Design review of the part built by this model. Coordinates are the model's own, in mm. A direction names the side the tool comes from. Give positions to 0.01 mm unless a question says otherwise; leave off trailing zeros. Loops run counter-clockwise (first coordinate to the right, second up) from the corner with the lowest first, then second, coordinate; pieces in that order, holes last. Notation, with made-up numbers: M 44,79 L 89,79 A19 ccw 89,103 Z; hole C -34,83.5 d2. An arc over 180 degrees is marked long. Answer as CSV lines item,"result".
```python
from build123d import *

# Parameters (mm, degrees)
SKETCH1_R                = 12.5
BOSS_EXTRUDE1_DEPTH      = 2.5
SKETCH2_R                = 1.35
CUT_EXTRUDE1_DEPTH       = 3.5
SKETCH4_R                = 2.1
CUT_EXTRUDE2_DEPTH       = 0.5
CUT_EXTRUDE3_DEPTH       = 3.5
FILLET3_R                = 1.6
CIRPATTERN1_COUNT        = 4
FILLET3_OF_CIRPATTERN1_R = 1.6
SKETCH3_R                = 1.45
BOSS_EXTRUDE2_DEPTH      = 6
FILLET2_R                = 2
SKETCH6_W                = 1.469693846
SKETCH6_H                = 0.4
SKETCH6_W_2              = 0.4
SKETCH6_H_2              = 1.469693846
CUT_EXTRUDE4_DEPTH       = 4


with BuildPart() as part:
    # Sketch1 → Boss-Extrude1 (new body)
    with BuildSketch(Plane(origin=(0, 0, 0), x_dir=(1, 0, 0), z_dir=(0, 1, 0))):
        Circle(SKETCH1_R)
    extrude(amount=BOSS_EXTRUDE1_DEPTH)

    # Sketch2 → Cut-Extrude1 (cut, through all)
    with BuildSketch(Plane(origin=(0, 2.5, 0), x_dir=(1, 0, 0), z_dir=(0, 1, 0))):
        with Locations((0, 9.5)):
            Circle(SKETCH2_R)
    cut_extrude1 = extrude(amount=-CUT_EXTRUDE1_DEPTH, mode=Mode.SUBTRACT)

    # Sketch4 → Cut-Extrude2 (cut)
    with BuildSketch(Plane(origin=(0, 2.5, 0), x_dir=(1, 0, 0), z_dir=(0, 1, 0))):
        with Locations((0, 9.5)):
            Circle(SKETCH4_R)
    cut_extrude2 = extrude(amount=-CUT_EXTRUDE2_DEPTH, mode=Mode.SUBTRACT)

    # Sketch5 → Cut-Extrude3 (cut, through all)
    with BuildSketch(Plane(origin=(0, 2.5, 0), x_dir=(1, 0, 0), z_dir=(0, 1, 0))):
        with BuildLine():
            Line((1.913417162, 4.619397663), (3.826834324, 9.238795325))
            ThreePointArc((3.826834324, 9.238795325), (7.071067812, 7.071067812), (9.238795325, 3.826834324))
            Line((9.238795325, 3.826834324), (4.619397663, 1.913417162))
            ThreePointArc((4.619397663, 1.913417162), (3.535533906, 3.535533906), (1.913417162, 4.619397663))
        make_face()
    cut_extrude3 = extrude(amount=-CUT_EXTRUDE3_DEPTH, mode=Mode.SUBTRACT)

    # Fillet3
    fillet3_edges = [part.edges().sort_by_distance(p)[0] for p in [
        (3.826834324, 1.25, -9.238795325),
        (9.238795325, 1.25, -3.826834324),
        (4.619397663, 1.25, -1.913417162),
        (1.913417162, 1.25, -4.619397663),
    ]]
    fillet(fillet3_edges, radius=FILLET3_R)

    # CirPattern1: Cut-Extrude1, Cut-Extrude2, Cut-Extrude3 ×4 about axis
    cirpattern1_axis = Axis((0, 0, 0), (0, 1, 0))
    for i in range(1, CIRPATTERN1_COUNT):
        add(cut_extrude1.rotate(cirpattern1_axis, i * 360 / CIRPATTERN1_COUNT), mode=Mode.SUBTRACT)
        add(cut_extrude2.rotate(cirpattern1_axis, i * 360 / CIRPATTERN1_COUNT), mode=Mode.SUBTRACT)
        add(cut_extrude3.rotate(cirpattern1_axis, i * 360 / CIRPATTERN1_COUNT), mode=Mode.SUBTRACT)

    # Fillet3 of CirPattern1
    fillet3_of_cirpattern1_edges = [part.edges().sort_by_distance(p)[0] for p in [
        (-9.238795325, 1.25, -3.826834324),
        (-3.826834324, 1.25, -9.238795325),
        (-1.913417162, 1.25, -4.619397663),
        (-4.619397663, 1.25, -1.913417162),
        (-3.826834324, 1.25, 9.238795325),
        (-9.238795325, 1.25, 3.826834324),
        (-4.619397663, 1.25, 1.913417162),
        (-1.913417162, 1.25, 4.619397663),
        (9.238795325, 1.25, 3.826834324),
        (3.826834324, 1.25, 9.238795325),
        (1.913417162, 1.25, 4.619397663),
        (4.619397663, 1.25, 1.913417162),
    ]]
    fillet(fillet3_of_cirpattern1_edges, radius=FILLET3_OF_CIRPATTERN1_R)

    # Sketch3 → Boss-Extrude2 (add)
    with BuildSketch(Plane(origin=(0, 2.5, 0), x_dir=(1, 0, 0), z_dir=(0, 1, 0))):
        Circle(SKETCH3_R)
    extrude(amount=BOSS_EXTRUDE2_DEPTH)

    # Fillet2
    fillet2_edges = [part.edges().sort_by_distance(p)[0] for p in [
        (-1.45, 2.5, 0),
    ]]
    fillet(fillet2_edges, radius=FILLET2_R)

    # Sketch6 → Cut-Extrude4 (cut)
    with BuildSketch(Plane(origin=(0, 8.5, 0), x_dir=(1, 0, 0), z_dir=(0, 1, 0))):
        with Locations((0, 1.45)):
            Rectangle(SKETCH6_W, SKETCH6_H)
        with Locations((-1.45, 0)):
            Rectangle(SKETCH6_W_2, SKETCH6_H_2)
    extrude(amount=-CUT_EXTRUDE4_DEPTH, mode=Mode.SUBTRACT)


solid = part.part
```
1. To check wall thickness, follow L1, parallel to X at y = 2.35, z = 0; L2, parallel to Z at x = 0, y = 1. State the ranges of each line that lie inside material, in increasing order. Write a range as [from, to].
Answer block:
L1,"[-12.5, -11.6], [-7.4, 7.4], [11.6, 12.5]"
L2,"[-12.5, -10.85], [-8.15, 8.15], [10.85, 12.5]"
2. We need section B-B, the plane x = 0. Write out the cut boundary in (y, z).
Answer block:
outline,"M 0,-12.5 L 2.5,-12.5 L 2.5,-11.6 L 2,-11.6 L 2,-10.85 L 0,-10.85 Z; M 0,-8.15 L 2,-8.15 L 2,-7.4 L 2.5,-7.4 L 2.5,-3.45 A2 cw 4.5,-1.45 L 4.5,-1.25 L 8.5,-1.25 L 8.5,1.45 L 4.5,1.45 A2 cw 2.5,3.45 L 2.5,7.4 L 2,7.4 L 2,8.15 L 0,8.15 Z; M 0,10.85 L 2,10.85 L 2,11.6 L 2.5,11.6 L 2.5,12.5 L 0,12.5 Z"
3. The part is to be moulded in two halves that separate along Z. For faces 3 (the cylindrical face through (-0.176, 1.014, -10.839)), 4 (the cylindrical face through (11.923, 1.232, -3.755)), 5 (the flat face through (-1.25, 7, 0)), say which applies: pulls with the +Z half, pulls with the -Z half, needs draft (parallel to the pull), parting line crosses it, or undercut.
Answer block:
face 3,"undercut"
face 4,"parting line crosses it"
face 5,"needs draft"
4. For faces 1 (the flat face through (-2.8, 1.27, 6.76)), 2 (the cylindrical face through (11.582, 2.254, -0.273)), list the 3-axis set-ups (+Z, -Z, +X, -X, +Y, -Y) from which the entire face can be reached by the end or side of a thin tool; tool diameter is ignored.
Answer block:
face 1,"+Y, -Y"
face 2,"+Y"
5. We need section C-C, the plane x = 9.5. Write out the cut boundary in (y, z).
Answer block:
outline,"M 0,-8.12 L 2.5,-8.12 L 2.5,-2.1 L 2,-2.1 L 2,-1.35 L 0,-1.35 Z; M 0,1.35 L 2,1.35 L 2,2.1 L 2.5,2.1 L 2.5,8.12 L 0,8.12 Z"
6. For P1, Ø6, axis at x = -7, z = -1, coming from the +Y side; P2, Ø5, axis at y = 6.5, z = 3.5, coming from the -X side; P3, Ø1.2, axis at y = 6, z = 0, coming from the -X side, all flat-tipped, find the tip position at first contact; note any pin that passes through.
Answer block:
P1,"y = 2.5"
P2,"x = -1.05"
P3,"x = -1.25"
7. We need section D-D, the plane y = 1. Count the separate pieces of the cut face and the enclosed holes in it, plus the area to 3 significant figures.
Answer block:
separate pieces,"1"
enclosed holes,"8"
area,"359 mm²"
8. We need section A-A, the plane z = 0. Write out the cut boundary in (x, y).
Answer block:
outline,"M -12.5,0 L -10.85,0 L -10.85,2 L -11.6,2 L -11.6,2.5 L -12.5,2.5 Z; M -8.15,0 L 8.15,0 L 8.15,2 L 7.4,2 L 7.4,2.5 L 3.45,2.5 A2 cw 1.45,4.5 L 1.45,8.5 L -1.25,8.5 L -1.25,4.5 L -1.45,4.5 A2 cw -3.45,2.5 L -7.4,2.5 L -7.4,2 L -8.15,2 Z; M 10.85,0 L 12.5,0 L 12.5,2.5 L 11.6,2.5 L 11.6,2 L 10.85,2 Z"
